from build123d import *

# Parameters (mm, degrees)
CROQUIS1_W              = 130
CROQUIS1_H              = 60
SALIENTE_EXTRUIR1_DEPTH = 7.5
CROQUIS1_4_W            = 150
CROQUIS1_4_H            = 80
CROQUIS1_4_W_2          = 130
CROQUIS1_4_H_2          = 60
SALIENTE_EXTRUIR2_DEPTH = 10


with BuildPart() as part:
    # Croquis1 → Saliente-Extruir1 (new body)
    with BuildSketch(Plane(origin=(0, 0, 0), x_dir=(1, 0, 0), z_dir=(0, 1, 0))):
        Rectangle(CROQUIS1_W, CROQUIS1_H)
    extrude(amount=-SALIENTE_EXTRUIR1_DEPTH)

    # Croquis1_4 → Saliente-Extruir2 (add)
    # profile 1 of 2: a face of its own
    with BuildSketch(Plane(origin=(0, 0, 0), x_dir=(1, 0, 0), z_dir=(0, 1, 0))):
        Rectangle(CROQUIS1_4_W, CROQUIS1_4_H)
        Rectangle(CROQUIS1_4_W_2, CROQUIS1_4_H_2, mode=Mode.SUBTRACT)
    # profile 2 of 2: a face of its own
    with BuildSketch(Plane(origin=(0, 0, 0), x_dir=(1, 0, 0), z_dir=(0, 1, 0))):
        Rectangle(CROQUIS1_4_W_2, CROQUIS1_4_H_2)
    extrude(amount=SALIENTE_EXTRUIR2_DEPTH)


solid = part.part
Work out the finished part from the listing and answer in its coordinate system (mm). A direction names the side the tool comes from. Give positions to 0.01 mm unless a question says otherwise; leave off trailing zeros. Loops run counter-clockwise (first coordinate to the right, second up) from the corner with the lowest first, then second, coordinate; pieces in that order, holes last. Notation, with made-up numbers: (12, 14.25) - (63, 14.25) arc R15 ccw to (63, 24.25) - close; hole circle Ø4 at (-8.75, 54.5). An arc over 180 degrees is marked (long way). Answer in a Markdown table with one row per item.
(1) Section A-A (z = -13.5) is taken. Give the vertices of the cut face in (x, y), and give its area (4 significant figures).
Results list:
| item | result |
|---|---|
| outline | (-75, 0) - (-65, 0) - (-65, -7.5) - (65, -7.5) - (65, 0) - (75, 0) - (75, 10) - (-75, 10) - close |
| area | 2,475 mm² |
(2) Section B-B (x = 59.5) is taken. Give the vertices of the cut face in (y, z).
Results list:
| item | result |
|---|---|
| outline | (-7.5, -30) - (0, -30) - (0, -40) - (10, -40) - (10, 40) - (0, 40) - (0, 30) - (-7.5, 30) - close |
(3) A tool of negligible diameter and unlimited length cuts with its end or side. For faces 1 (the face through (65, -4, 0)), 2 (the face through (-1, 10, -1)), 3 (the face through (-1, -4, -30)), 4 (the face through (-65, -4, 0)), 5 (the face through (-1, -4, 30)), from which of +Z, -Z, +X, -X, +Y, -Y can it reach the whole face along a straight path? Write none if from no direction.
Results list:
| item | result |
|---|---|
| face 1 | +Z, -Z, +X, -Y |
| face 2 | +Z, -Z, +X, -X, +Y |
| face 3 | -Z, +X, -X, -Y |
| face 4 | +Z, -Z, -X, -Y |
| face 5 | +Z, +X, -X, -Y |
(4) Flat-ended cylindrical pins translate along their axes: pin 1 Ø2 at (x, y) = (-16, -4) entering from +Z; pin 2 Ø4 at (y, z) = (-5, -3.5) entering from +X; pin 3 Ø4 at (y, z) = (-3, -14) entering from -X; pin 4 Ø6 at (y, z) = (-1, -3) entering from -X. Find the tip coordinate at first contact, or state that the pin passes through.
Results list:
| item | result |
|---|---|
| pin 1 | stops at z = 30 |
| pin 2 | stops at x = 65 |
| pin 3 | stops at x = -65 |
| pin 4 | stops at x = -75 |
(5) Consider L1, parallel to Y at x = -43, z = -35; L2, parallel to Z at x = -43.5, y = -6.5; L3, parallel to X at y = -2, z = -3. Determine where each line is inside the solid, lowest interval first. Write a range as [from, to].
Results list:
| item | result |
|---|---|
| L1 | y = [0, 10] |
| L2 | z = [-30, 30] |
| L3 | x = [-65, 65] |
(6) Section C-C (y = -2.5) is taken. Give the vertices of the cut face in (x, z).
Results list:
| item | result |
|---|---|
| outline | (-65, -30) - (65, -30) - (65, 30) - (-65, 30) - close |
